Autodesk Inventor part; units mm, degrees
ref_plane "YZ Plane" through (0, 0, 0) normal (1, 0, 0) x (0, 1, 0)
ref_plane "XZ Plane" through (0, 0, 0) normal (0, 1, 0) x (-1, 0, 0)
ref_plane "XY Plane" through (0, 0, 0) normal (0, 0, 1) x (1, 0, 0)
sketch "Sketch1" plane through (0, 0, 0) normal (0, 1, 0) x (-1, 0, 0)
  line L0 (-75, -425) -> (75, -425)
  line L1 (75, -425) -> (75, 425)
  line L2 (75, 425) -> (-75, 425)
  line L3 (-75, 425) -> (-75, -425)
  line L4 (-75, -425) -> (75, 425) construction
  line L5 (75, -425) -> (-75, 425) construction
  point P0 (0, 0)
  dimension "d0" = 850
  dimension "d1" = 150
extrude "Extrusion1" add sketch "Sketch1" along normal blind 18.55
sketch "Sketch2" plane through (0, 18.55, 0) normal (0, 1, 0) x (1, 0, 0)
  line L0 (18.55, -365) -> (-18.55, -365)
  line L1 (-18.55, -365) -> (-18.55, -340)
  line L2 (-18.55, -340) -> (18.55, -340)
  line L3 (18.55, -340) -> (18.55, -365)
  line L4 (18.55, -365) -> (-18.55, -340) construction
  line L5 (-18.55, -365) -> (18.55, -340) construction
  line L6 (18.55, 340) -> (-18.55, 340)
  line L7 (-18.55, 340) -> (-18.55, 365)
  line L8 (-18.55, 365) -> (18.55, 365)
  line L9 (18.55, 365) -> (18.55, 340)
  line L10 (18.55, 340) -> (-18.55, 365) construction
  line L11 (-18.55, 340) -> (18.55, 365) construction
  line L12 (0, -365) -> (0, -425) construction
  line L13 (-75, -425) -> (75, -425)
  line L14 (0, 365) -> (0, 425) construction
  line L15 (75, 425) -> (-75, 425)
  point P0 (0, 0)
  point P1 (0, -352.5)
  point P2 (0, 352.5)
  dimension "d4" = 730
  dimension "d5" = 25
  dimension "d6" = 37.1
extrude "Extrusion2" cut sketch "Sketch2" against normal blind 18.55
properties part number "floor_Part"
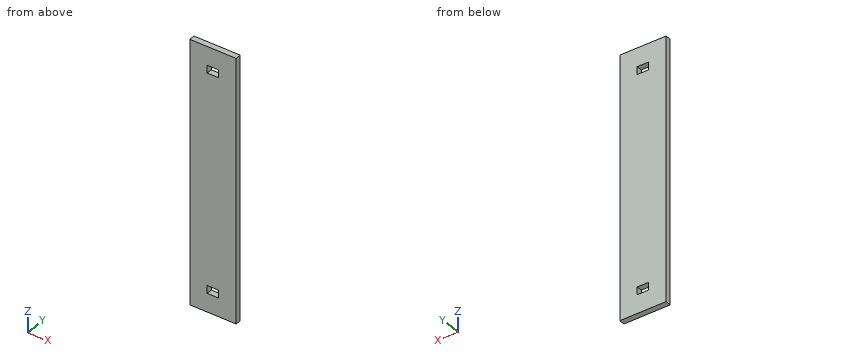
Work out the finished part from the listing and answer in its coordinate system (mm). Give positions to 0.01 mm unless a question says otherwise; leave off trailing zeros. Order: outer loops, then holes, each group sorted by start corner. A loop starts at its lowest first (then second) coordinate and runs counter-clockwise, first axis right, second up. Notation, with made-up numbers: (75, 13) - (109, 13) arc R20 ccw to (109, 46) - close; hole circle Ø3 at (84.25, 15.25). An arc over 180 degrees is marked (long way). Answer as CSV lines item,"result". Start each with the question number.
Q1. Given pin 1 Ø1.5 at (x, z) = (9, 109) entering from -Y, flat-ended and moving along its own axis, determine where the tip first touches the part or whether it passes through.
Q2. Find the intervals of material crossed by L1, parallel to Z at x = 9, y = 3.75; L2, parallel to X at y = 11, z = -343, in increasing order. Write a range as [from, to].
Q3. The part is cut by section A-A (x = -7). Write down the section's boundary in (y, z), then the cut area to 3 significant figures.
Check result:
1,pin 1,"stops at y = 0"
2,L1,"z = [-425, -365], [-340, 340], [365, 425]"
2,L2,"x = [-75, -18.55], [18.55, 75]"
3,outline,"(0, -425) - (18.55, -425) - (18.55, -365) - (0, -365) - close; (0, -340) - (18.55, -340) - (18.55, 340) - (0, 340) - close; (0, 365) - (18.55, 365) - (18.55, 425) - (0, 425) - close"
3,area,"14,800 mm²"
